The model under review builds one solid part; all positions refer to its coordinate system, in mm. Face numbers are marked on the shaded views. A direction names the side the tool comes from. Round coordinates to 2 decimals unless told otherwise and drop trailing zeros. Loops run counter-clockwise (first coordinate to the right, second up) from the corner with the lowest first, then second, coordinate; pieces in that order, holes last. Notation, with made-up numbers: M 21.25,-20 L 61.25,-20 A25 cw 61.25,-7 Z; hole C -28,-38 d5. An arc over 180 degrees is marked long. Return JSON: item names as keys, results as strings. Group by question number.
Q1. Consider section B-B (y = -11.75). State the section outline as (x, z) points.
Q2. Draft analysis for pull direction X (two halves, no side actions). For the marked faces 4, 5 and 6, state which applies: pulls with the +X half, pulls with the -X half, needs draft (parallel to the pull), parting line crosses it, or undercut.
Q3. Clearance check with flat-ended pins moving along their axes: pin 1 Ø6 at (y, z) = (7, 7) entering from +X; pin 2 Ø1.5 at (x, z) = (2.5, 11) entering from +Y; pin 3 Ø6.5 at (x, z) = (7, 13) entering from +Y. State where each tip first meets the part, or that it passes through.
Q4. Consider section C-C (x = -3.25). State the section outline as (y, z) points.
Q5. To check wall thickness, follow line 1 along X through (y, z) = (-0.25, 4); line 2 along Y through (x, z) = (0.25, 11.25); line 3 along X through (y, z) = (1, 15.5). State the ranges of each line that lie inside material, in increasing order.
Q6. For the marked faces 1, 2 and 3, list the 3-axis set-ups (+Z, -Z, +X, -X, +Y, -Y) from which the entire face can be reached by the end or side of a thin tool; tool diameter is ignored.
from build123d import *

# Parameters (mm, degrees)
PAD_DEPTH   = 20
FILLET_R    = 12
FILLET001_R = 11.99
FILLET002_R = 7.99


with BuildPart() as part:
    # Sketch → Pad (new body)
    with BuildSketch(Plane.XY):
        Polygon((-12, 10), (-4, 10), (-4, -4), (4, -4), (4, 0), (12, 0), (12, -15), (-12, -15), align=None)
    extrude(amount=PAD_DEPTH)

    # Fillet
    fillet_edges = [part.edges().sort_by_distance(p)[0] for p in [
        (-12, -15, 10),
    ]]
    fillet(fillet_edges, radius=FILLET_R)

    # Fillet001
    fillet001_edges = [part.edges().sort_by_distance(p)[0] for p in [
        (12, -15, 10),
    ]]
    fillet(fillet001_edges, radius=FILLET001_R)

    # Fillet002
    fillet002_edges = [part.edges().sort_by_distance(p)[0] for p in [
        (-12, 10, 10),
    ]]
    fillet(fillet002_edges, radius=FILLET002_R)


solid = part.part
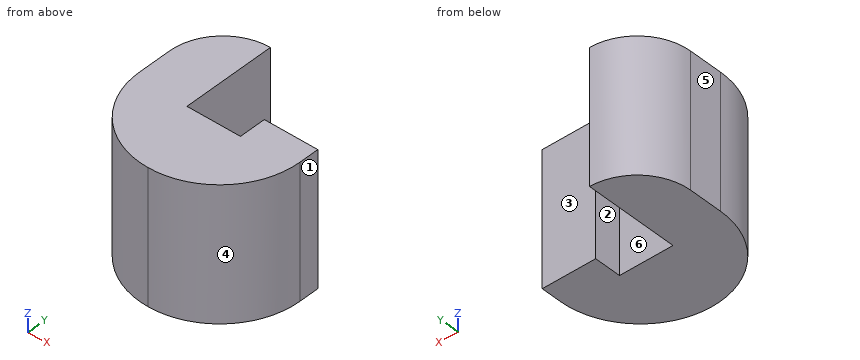
Values:
{
 "1": {"outline": "M -8.21,0 L 8.22,0 L 8.22,20 L -8.21,20 Z"},
 "2": {"face 4": "pulls with the +X half", "face 5": "pulls with the -X half", "face 6": "undercut"},
 "3": {"pin 1": "stops at x = -4", "pin 2": "stops at y = -4", "pin 3": "stops at y = 0"},
 "4": {"outline": "M -14.55,0 L -4,0 L -4,20 L -14.55,20 Z"},
 "5": {"line 1": "x = -12 to -4, 4 to 12", "line 2": "y = -15 to -4", "line 3": "x = -12 to -4"},
 "6": {"face 1": "+Z, -Z, +X, +Y, -Y", "face 2": "+Z, -Z, +Y", "face 3": "+Z, -Z, +X, +Y"}
}
